Verification items for the finished model (mm, model axes). Face numbers are marked on the shaded views. Give positions to 0.01 mm unless a question says otherwise; leave off trailing zeros. Write each loop counter-clockwise with the first axis right and the second up, starting at its lowest first coordinate (ties: lowest second). Pieces come first, ordered by that corner, then holes.
Autodesk Inventor part; units mm, degrees
ref_plane "YZ Plane" through (0, 0, 0) normal (1, 0, 0) x (0, 1, 0)
ref_plane "XZ Plane" through (0, 0, 0) normal (0, 1, 0) x (-1, 0, 0)
ref_plane "XY Plane" through (0, 0, 0) normal (0, 0, 1) x (1, 0, 0)
ref_plane "Work Plane1" through (0, 0, 0) normal (0, 0, 1) x (1, 0, 0)
sketch "Sketch1" plane through (0, 0, 0) normal (0, 0, 1) x (1, 0, 0)
  point P0 (0, 0)
ref_plane "Work Plane2" through (0, 0, 0) normal (0, 0, 1) x (1, 0, 0)
sketch "Sketch2" plane through (0, 0, 0) normal (0, 0, 1) x (1, 0, 0)
  line L0 (133.9999, 0) -> (0, 0) construction
  line L1 (133.9999, 0) -> (133.9999, 2) construction
  line L2 (0, 2) -> (133.9999, 2) construction
  line L3 (0, 0) -> (0, 2) construction
  line L4 (137.0698, 41) -> (137.0698, 2)
  line L5 (137.0698, 2) -> (-2.9302, 2)
  line L6 (-2.9302, 2) -> (-2.9302, 41)
  line L7 (-2.9302, 47) -> (137.0698, 2) construction
  line L8 (137.0698, 47) -> (-2.9302, 2) construction
  line L9 (22.0698, 29) -> (112.0698, 29)
  line L10 (22.0698, 29) -> (13.7788, 44.8537)
  line L11 (67.0698, 29) -> (67.0698, 47) construction
  line L12 (112.0698, 29) -> (120.3608, 44.8537)
  line L13 (3.0698, 47) -> (10.2342, 47)
  line L14 (123.9053, 47) -> (131.0698, 47)
  arc A0 (13.7788, 44.8537) -> (10.2342, 47) centre (10.2342, 43) ccw
  arc A1 (123.9053, 47) -> (120.3608, 44.8537) centre (123.9053, 43) ccw
  arc A2 (3.0698, 47) -> (-2.9302, 41) centre (3.0698, 41) ccw
  arc A3 (137.0698, 41) -> (131.0698, 47) centre (131.0698, 41) ccw
  circle A4 centre (6.8088, 39) radius 4
  circle A5 centre (127.3308, 39) radius 4
  point P0 (67.0698, 24.5)
  point P1 (12.6563, 47)
  point P2 (121.4832, 47)
  dimension "d0" = 140
  dimension "d1" = 45
  dimension "d6" = 25
  dimension "d7" = 25
  dimension "d8" = 4
  dimension "d9" = 6
  dimension "d10" = 45
  dimension "d11" = 8
  dimension "d12" = 8
  dimension "d16" = 120.522
extrude "Extrusion1" add sketch "Sketch2" against normal blind 10
properties part number "supporto_guide_lungo"
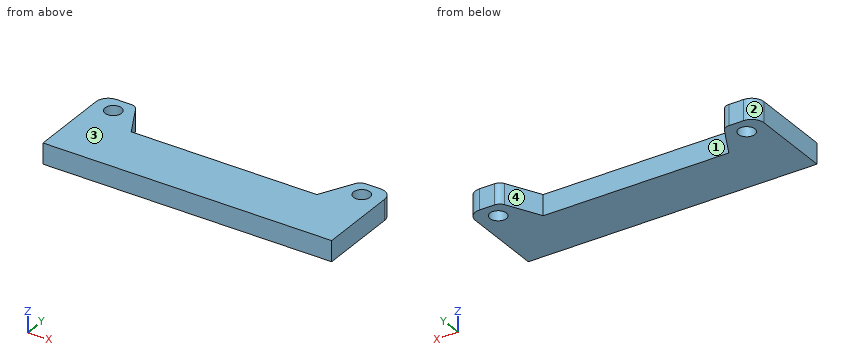
Item 1: Release check for a two-part mould opening along X. For the marked faces 1, 2, 3 and 4 record: released by +X, released by -X, zero draft, split by the parting line, or undercut.
Answer key:
face 1: undercut
face 2: released by -X
face 3: zero draft
face 4: undercut
Item 2: Sectioned sample at B-B on y = 39. Record the cut outline in (x, z).
Answer key:
outline: (-2.93, -10) - (2.81, -10) - (2.81, 0) - (-2.93, 0) - close; (10.81, -10) - (16.84, -10) - (16.84, 0) - (10.81, 0) - close; (117.3, -10) - (123.33, -10) - (123.33, 0) - (117.3, 0) - close; (131.33, -10) - (137.07, -10) - (137.07, 0) - (131.33, 0) - close
Item 3: Sectioned sample at D-D on x = 114.5. Record the cut outline in (y, z), then the cut area to 3 significant figures.
Answer key:
outline: (2, -10) - (33.65, -10) - (33.65, 0) - (2, 0) - close
area: 316 mm2
Item 4: Sectioned sample at C-C on x = 54.5. Record the cut outline in (y, z).
Answer key:
outline: (2, -10) - (29, -10) - (29, 0) - (2, 0) - close
Item 5: Sectioned sample at A-A on z = -8.75. Record the cut outline in (x, y).
Answer key:
outline: (-2.93, 2) - (137.07, 2) - (137.07, 41) arc R6 ccw to (131.07, 47) - (123.91, 47) arc R4 ccw to (120.36, 44.85) - (112.07, 29) - (22.07, 29) - (13.78, 44.85) arc R4 ccw to (10.23, 47) - (3.07, 47) arc R6 ccw to (-2.93, 41) - close; hole circle Ø8 at (6.81, 39); hole circle Ø8 at (127.33, 39)
Item 6: Scan lines: line 1 along Y through (x, z) = (127.5, -3.25); line 2 along Y through (x, z) = (128.5, -3.5); line 3 along X through (y, z) = (42.5, -1.5). Record each from-to range of solid material in increasing order.
Answer key:
line 1: y = 2 to 35, 43 to 47
line 2: y = 2 to 35.17, 42.83 to 47
line 3: x = -2.74 to 4.87, 8.75 to 15.01, 119.13 to 125.39, 129.27 to 136.88
Item 7: Depth check by flat-ended pin: pin 1 (13 mm diameter, centred on x = 6.81, y = 39, fed in from -Z); pin 2 (3 mm diameter, centred on x = 105, z = -5.5, fed in from +Y). Enter the tip coordinate at first touch or a pass-through.
Answer key:
pin 1: stops at z = -10
pin 2: stops at y = 29
